Build history of the part. All positions in model axes, mm. Round coordinates to 2 decimals unless told otherwise and drop trailing zeros. Write each loop counter-clockwise with the first axis right and the second up, starting at its lowest first coordinate (ties: lowest second). Pieces come first, ordered by that corner, then holes. Notation, with made-up numbers: M 51.25,-3 L 100.25,-3 A19 cw 100.25,6 Z; hole C 50.25,67 d3. An arc over 180 degrees is marked long. Use a Markdown table: item, result.
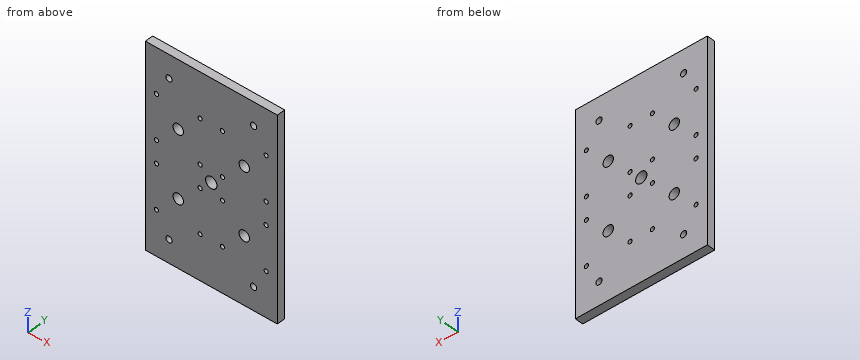
from build123d import *

# Parameters (mm, degrees)
SKETCH1_W           = 101.6
SKETCH1_H           = 152.4
SKETCH1_R           = 4
SKETCH1_R_2         = 1.5875
SKETCH1_R_3         = 4.365625
SKETCH1_R_4         = 2.38125
BOSS_EXTRUDE1_DEPTH = 6.35


with BuildPart() as part:
    # Sketch1 → Boss-Extrude1 (new body)
    with BuildSketch(Plane(origin=(0, 0, 0), x_dir=(1, 0, 0), z_dir=(0, 1, 0))):
        Rectangle(SKETCH1_W, SKETCH1_H)
        with Locations(Location((-25.4, 25.4, 0), (0, 0, 270))):
            Circle(SKETCH1_R, mode=Mode.SUBTRACT)
        with Locations(Location((-42.225, 42.225, 0), (0, 0, 270))):
            Circle(SKETCH1_R_2, mode=Mode.SUBTRACT)
        with Locations(Location((-8.575, 42.225, 0), (0, 0, 90))):
            Circle(SKETCH1_R_2, mode=Mode.SUBTRACT)
        with Locations(Location((-8.575, 8.575, 0), (0, 0, 270))):
            Circle(SKETCH1_R_2, mode=Mode.SUBTRACT)
        with Locations(Location((-42.225, 8.575, 0), (0, 0, 90))):
            Circle(SKETCH1_R_2, mode=Mode.SUBTRACT)
        with Locations(Location((8.575, 8.575, 0), (0, 0, 90))):
            Circle(SKETCH1_R_2, mode=Mode.SUBTRACT)
        with Locations(Location((42.225, 8.575, 0), (0, 0, 270))):
            Circle(SKETCH1_R_2, mode=Mode.SUBTRACT)
        with Locations(Location((42.225, 42.225, 0), (0, 0, 90))):
            Circle(SKETCH1_R_2, mode=Mode.SUBTRACT)
        with Locations(Location((8.575, 42.225, 0), (0, 0, 270))):
            Circle(SKETCH1_R_2, mode=Mode.SUBTRACT)
        with Locations(Location((25.4, 25.4, 0), (0, 0, 90))):
            Circle(SKETCH1_R, mode=Mode.SUBTRACT)
        with Locations(Location((42.225, -8.575, 0), (0, 0, 90))):
            Circle(SKETCH1_R_2, mode=Mode.SUBTRACT)
        with Locations(Location((42.225, -42.225, 0), (0, 0, 270))):
            Circle(SKETCH1_R_2, mode=Mode.SUBTRACT)
        with Locations(Location((8.575, -42.225, 0), (0, 0, 90))):
            Circle(SKETCH1_R_2, mode=Mode.SUBTRACT)
        with Locations(Location((25.4, -25.4, 0), (0, 0, 270))):
            Circle(SKETCH1_R, mode=Mode.SUBTRACT)
        with Locations(Location((8.575, -8.575, 0), (0, 0, 270))):
            Circle(SKETCH1_R_2, mode=Mode.SUBTRACT)
        with Locations(Location((-8.575, -8.575, 0), (0, 0, 90))):
            Circle(SKETCH1_R_2, mode=Mode.SUBTRACT)
        with Locations(Location((-42.225, -8.575, 0), (0, 0, 270))):
            Circle(SKETCH1_R_2, mode=Mode.SUBTRACT)
        with Locations(Location((-8.575, -42.225, 0), (0, 0, 270))):
            Circle(SKETCH1_R_2, mode=Mode.SUBTRACT)
        with Locations(Location((-25.4, -25.4, 0), (0, 0, 90))):
            Circle(SKETCH1_R, mode=Mode.SUBTRACT)
        with Locations(Location((-42.225, -42.225, 0), (0, 0, 90))):
            Circle(SKETCH1_R_2, mode=Mode.SUBTRACT)
        with Locations(Location((0, 0, 0), (0, 0, 270))):
            Circle(SKETCH1_R_3, mode=Mode.SUBTRACT)
        with Locations(Location((32.54375, 58.7375, 0), (0, 0, 270))):
            Circle(SKETCH1_R_4, mode=Mode.SUBTRACT)
        with Locations(Location((32.54375, -58.7375, 0), (0, 0, 90))):
            Circle(SKETCH1_R_4, mode=Mode.SUBTRACT)
        with Locations(Location((-32.54375, -58.7375, 0), (0, 0, 270))):
            Circle(SKETCH1_R_4, mode=Mode.SUBTRACT)
        with Locations(Location((-32.54375, 58.7375, 0), (0, 0, 90))):
            Circle(SKETCH1_R_4, mode=Mode.SUBTRACT)
    extrude(amount=BOSS_EXTRUDE1_DEPTH)


solid = part.part
Q1. Cut at B-B on z = 0. Give the cut face in (x, y), and give its area (3 significant figures).
Response values:
| item | result |
|---|---|
| outline | M -50.8,0 L -4.37,0 L -4.37,6.35 L -50.8,6.35 Z; M 4.37,0 L 50.8,0 L 50.8,6.35 L 4.37,6.35 Z |
| area | 590 mm2 |
Q2. Cut at A-A on x = 0. Give the cut face in (y, z), and give its area (3 significant figures).
Response values:
| item | result |
|---|---|
| outline | M 0,-76.2 L 6.35,-76.2 L 6.35,-4.37 L 0,-4.37 Z; M 0,4.37 L 6.35,4.37 L 6.35,76.2 L 0,76.2 Z |
| area | 912 mm2 |
Q3. Cut at C-C on z = -25.4. Give the cut face in (x, y), and give its area (3 significant figures).
Response values:
| item | result |
|---|---|
| outline | M -50.8,0 L -29.4,0 L -29.4,6.35 L -50.8,6.35 Z; M -21.4,0 L 21.4,0 L 21.4,6.35 L -21.4,6.35 Z; M 29.4,0 L 50.8,0 L 50.8,6.35 L 29.4,6.35 Z |
| area | 544 mm2 |
Q4. Drill centre lines: L1, parallel to X at y = 2.75, z = 25.4; L2, parallel to X at y = 4.5, z = 0; L3, parallel to X at y = 6, z = 58. Where is each one in solid material? Low to high.
Response values:
| item | result |
|---|---|
| L1 | x = -50.8 to -29.4, -21.4 to 21.4, 29.4 to 50.8 |
| L2 | x = -50.8 to -4.37, 4.37 to 50.8 |
| L3 | x = -50.8 to -34.81, -30.28 to 30.28, 34.81 to 50.8 |
Q5. Cut at D-D on y = 3.5. Count the separate pieces of the cut face and the enclosed holes in it, and give its area (3 significant figures).
Response values:
| item | result |
|---|---|
| separate pieces | 1 |
| enclosed holes | 25 |
| area | 15,000 mm2 |
